```python
from build123d import *

# Parameters (mm, degrees)
SKETCH1_W           = 20
SKETCH1_H           = 20
SKETCH1_R           = 1.5
BOSS_EXTRUDE1_DEPTH = 3
SKETCH2_W           = 20
SKETCH2_H           = 3
BOSS_EXTRUDE2_DEPTH = 17
SKETCH3_R           = 1.5
CUT_EXTRUDE1_DEPTH  = 30
BOSS_EXTRUDE3_DEPTH = 3
BOSS_EXTRUDE4_START = -20
BOSS_EXTRUDE4_DEPTH = 3


with BuildPart() as part:
    # Sketch1 → Boss-Extrude1 (new body)
    with BuildSketch(Plane(origin=(0, 0, 0), x_dir=(1, 0, 0), z_dir=(0, 1, 0))):
        Rectangle(SKETCH1_W, SKETCH1_H)
        with Locations(Location((-4.242640687, 4.242640687, 0), (0, 0, 270))):
            Circle(SKETCH1_R, mode=Mode.SUBTRACT)
        with Locations(Location((4.242640687, -4.242640687, 0), (0, 0, 270))):
            Circle(SKETCH1_R, mode=Mode.SUBTRACT)
    extrude(amount=BOSS_EXTRUDE1_DEPTH)

    # Sketch2 → Boss-Extrude2 (add)
    with BuildSketch(Plane(origin=(0, 3, 0), x_dir=(1, 0, 0), z_dir=(0, 1, 0))):
        with Locations((0, 8.5)):
            Rectangle(SKETCH2_W, SKETCH2_H)
    extrude(amount=BOSS_EXTRUDE2_DEPTH)

    # Sketch3 → Cut-Extrude1 (cut)
    with BuildSketch(Plane(origin=(0, 0, -10), x_dir=(-1, 0, 0), z_dir=(0, 0, -1))):
        with Locations((-4.242640687, 14.242640687)):
            Circle(SKETCH3_R)
        with Locations((4.242640687, 5.757359313)):
            Circle(SKETCH3_R)
    extrude(amount=-CUT_EXTRUDE1_DEPTH, mode=Mode.SUBTRACT)

    # Sketch4 → Boss-Extrude3 (add)
    with BuildSketch(Plane.ZY.offset(10)):
        Polygon((-7, 11.5), (1.5, 3), (-7, 3), align=None)
    extrude(amount=-BOSS_EXTRUDE3_DEPTH)

    # Sketch4<2> → Boss-Extrude4 (add)
    with BuildSketch(Plane.ZY.offset(10).offset(BOSS_EXTRUDE4_START)):
        Polygon((-7, 11.5), (1.5, 3), (-7, 3), align=None)
    extrude(amount=BOSS_EXTRUDE4_DEPTH)


solid = part.part
```
Could you check a few things on this model? Use its own coordinates, in mm. A direction names the side the tool comes from. Give positions to 0.01 mm unless a question says otherwise; leave off trailing zeros. Order: outer loops, then holes, each group sorted by start corner. A loop starts at its lowest first (then second) coordinate and runs counter-clockwise, first axis right, second up.
Q1. We'd pull the mould along X, two halves only. Please class faces 3 (the flat face through (-10, 6, -4)), 4 (the flat face through (10, 6, -4)), 5 (the flat face through (0, 1, 10)), 6 (the cylindrical face through (4.57, 12.78, -8.52)): +X half, -X half, draft (parallel to the pull), parting line (faces both ways), or undercut.
Q2. Suppose I cut it at C-C, the plane y = 1.5. Write out the boundary of the cut face in (x, z).
Q3. If I drill on line 1 along Y through (x, z) = (3, -2.5); line 2 along Z through (x, y) = (-6, 8.75); line 3 along Y through (x, z) = (3.5, -8.5), over which ranges is the centre line in solid material (lowest first)?
Q4. I'm going to push flat-ended pins straight in: P1, Ø1.8, axis at x = 4.24, y = 14.24, coming from the +Z side; P2, Ø1.5, axis at x = -3.5, y = 15, coming from the +Z side. Where does each tip first touch, or does it pass through?
Q5. Suppose I cut it at B-B, the plane z = -5.25. Write out the boundary of the cut face in (x, y), and give its area (3 significant figures).
Q6. Suppose I cut it at A-A, the plane z = 0.75. Write out the boundary of the cut face in (x, y).
Q7. For faces 1 (the flat face through (7, 5, -5)), 2 (the flat face through (8.5, 7.3, -2.8)), which set-ups out of +Z, -Z, +X, -X, +Y, -Y let a thin tool reach every point of the face, with its end or its side?
Q8. Suppose I cut it at D-D, the plane x = -8.5. Write out the boundary of the cut face in (y, z), and give its area (3 significant figures).
Solution:
1. face 3: -X half
1. face 4: +X half
1. face 5: draft
1. face 6: undercut
2. outline: (-10, -10) - (10, -10) - (10, 10) - (-10, 10) - close; hole circle Ø3 at (-4.24, -4.24); hole circle Ø3 at (4.24, 4.24)
3. line 1: y = 0 to 3
3. line 2: z = -10 to -7
3. line 3: y = 0 to 12.94, 15.55 to 20
4. P1: passes through
4. P2: stops at z = -7
5. outline: (-10, 0) - (-5.35, 0) - (-5.35, 3) - (-7, 3) - (-7, 9.75) - (-10, 9.75) - close; (-3.13, 0) - (10, 0) - (10, 9.75) - (7, 9.75) - (7, 3) - (-3.13, 3) - close
5. area: 93.8 mm2
6. outline: (-10, 0) - (10, 0) - (10, 3.75) - (7, 3.75) - (7, 3) - (-7, 3) - (-7, 3.75) - (-10, 3.75) - close
7. face 1: +Z, +Y
7. face 2: +Z, +X, -X, +Y
8. outline: (0, -10) - (20, -10) - (20, -7) - (11.5, -7) - (3, 1.5) - (3, 10) - (0, 10) - close
8. area: 147 mm2
